from build123d import *

# Parameters (mm, degrees)
SKETCH2_R                 = 1.5
MAIN_EXTRUDE_DEPTH        = 21.5
HORIZONTAL_CUT_DEPTH      = 48.59062889
HORIZONTAL_CUT_DEPTH_BACK = 48.59062889
SKETCH5_OUTSIDE_W         = 47.542
SKETCH5_OUTSIDE_H         = 58.496
VERTICAL_CUT_DEPTH        = 15.063100578
END_FILLET_R              = 2
SPRING_PLACE_CUT_DEPTH    = 14
FILLET5_R                 = 10
FILLET4_R                 = 5
CUT_EXTRUDE1_DEPTH        = 52.882041504
CUT_EXTRUDE2_START        = -16.243126
CUT_EXTRUDE2_DEPTH        = 16.243126


# Read off the part's stored shape, not the designer's step: vertical-cut
with BuildPart() as part:
    # Sketch2 → main-extrude (new, symmetric)
    with BuildSketch(Plane.XY):
        with BuildLine():
            Line((26.046045858, 30.659682992), (19.902405526, 34.961506265))
            Line((19.902405526, 34.961506265), (11.298758981, 22.6742256))
            Line((11.298758981, 22.6742256), (1.690473047, 27.154642913))
            ThreePointArc((1.690473047, 27.154642913), (-2.003746596, 26.991347579), (-3.985523805, 23.869411765))
            Line((-3.985523805, 23.869411765), (-5.978285707, 0.51))
            ThreePointArc((-5.978285707, 0.51), (-1.419809226, -5.829591904), (5.543277195, -2.296100594))
            Line((5.543277195, -2.296100594), (7.669311717, -2.952527164))
            Line((7.669311717, -2.952527164), (7.722039638, 4.490290033))
            Line((7.722039638, 4.490290033), (26.046045858, 30.659682992))
        make_face()
        Circle(SKETCH2_R, mode=Mode.SUBTRACT)
        with Locations((0, 23.529411765)):
            Circle(SKETCH2_R, mode=Mode.SUBTRACT)
    extrude(amount=MAIN_EXTRUDE_DEPTH, both=True)

    # Sketch5 outside → horizontal-cut (cut, two sides: drawn at the far end of the back side and taken through both)
    with BuildSketch(Plane(origin=(0, 27.529411765, 0), x_dir=(-1, 0, 0), z_dir=(0, -1, 0)).offset(-HORIZONTAL_CUT_DEPTH_BACK)):
        with Locations((-10.023, 0)):
            Rectangle(SKETCH5_OUTSIDE_W, SKETCH5_OUTSIDE_H)
        Polygon((-5.543277195, -21.5), (6, -21.5), (6, 21.5), (-5.543277195, 21.5), (-7.669311717, 21.5), (-11.298758981, 7.5), (-26.046045858, 7.5), (-26.046045858, -7.5), (-11.298758981, -7.5), (-7.669311717, -21.5), align=None, mode=Mode.SUBTRACT)
    extrude(amount=HORIZONTAL_CUT_DEPTH + HORIZONTAL_CUT_DEPTH_BACK, mode=Mode.SUBTRACT)

    # vertical-cut outline → vertical-cut (cut)
    with BuildSketch(Plane(origin=(-1.956623805, 47.652438964, 0), x_dir=(0, 0, 1), z_dir=(0.9963809512430475, -0.08499999999999992, 0))):
        Polygon((10, 28.250815058), (10, 18), (21.5, 18), (21.5, 41.313669441), align=None)
        Polygon((-21.5, 18), (-10, 18), (-10, 28.250815058), (-21.5, 41.313669441), align=None)
    extrude(amount=VERTICAL_CUT_DEPTH, mode=Mode.SUBTRACT)

    # end-fillet
    end_fillet_edges = [part.edges().sort_by_distance(p)[0] for p in [
        (19.902405526, 34.961506265, 0),
        (26.046045858, 30.659682992, 0),
        (22.974225692, 32.810594628, 7.5),
        (22.974225692, 32.810594628, -7.5),
    ]]
    fillet(end_fillet_edges, radius=END_FILLET_R)

    # Sketch13 → spring-place-cut (cut, symmetric)
    with BuildSketch(Plane.XY):
        with BuildLine():
            Line((4.750311853, 13.645607612), (-4.788285707, 14.459333317))
            Line((-4.788285707, 14.459333317), (-5.468285707, 6.488285707))
            Line((-5.468285707, 6.488285707), (-5.978285707, 0.51))
            ThreePointArc((-5.978285707, 0.51), (-1.419809226, -5.829591904), (5.543277195, -2.296100594))
            Line((5.543277195, -2.296100594), (5.568173284, -2.303787419))
            Line((5.568173284, -2.303787419), (5.732956787, -1.770086573))
            ThreePointArc((5.732956787, -1.770086573), (5.96812639, -0.61763047), (5.973944242, 0.558560826))
            Line((5.973944242, 0.558560826), (4.750311853, 13.645607612))
        make_face()
    extrude(amount=SPRING_PLACE_CUT_DEPTH, both=True, mode=Mode.SUBTRACT)

    # Fillet5
    fillet5_edges = [part.edges().sort_by_distance(p)[0] for p in [
        (-0.018986927, 14.052470465, 14),
        (-0.018986927, 14.052470465, -14),
    ]]
    fillet(fillet5_edges, radius=FILLET5_R)

    # Fillet4
    # the kernel refuses this fillet: 5 mm, written as the material it adds along each edge
    with BuildSketch(Plane(origin=(11.298758981, 22.6742256, -17.98874539), x_dir=(-0.9063077870366477, 0.42261826174070405, 0), z_dir=(0, 0, 1))) as fillet4_piece_1_section:
        with BuildLine():
            CenterArc((FILLET4_R * 0.839099631177, -FILLET4_R), FILLET4_R, 90, 80)
            Line((-FILLET4_R * 0.145708121835, -FILLET4_R * 0.826351822333), (0, 0))
            Line((0, 0), (FILLET4_R * 0.839099631177, 0))
        make_face()
    fillet4_piece_1 = extrude(amount=25.48874539, mode=Mode.PRIVATE)
    fillet4_piece_1 = split(fillet4_piece_1, bisect_by=Plane(origin=(9.938648559, 23.630642265, -10), z_dir=(0, 0, 1)), keep=Keep.TOP, mode=Mode.PRIVATE)
    fillet4_piece_1 = split(fillet4_piece_1, bisect_by=Plane(origin=(10.933336463, 23.630642265, -8.909557674), z_dir=(-0.9679999612731994, 0, 0.25095034364408525)), keep=Keep.TOP, mode=Mode.PRIVATE)
    fillet4_piece_1 = split(fillet4_piece_1, bisect_by=Plane(origin=(9.938648559, 23.630642265, -7.5), z_dir=(0, 0, -1)), keep=Keep.TOP, mode=Mode.PRIVATE)
    add(fillet4_piece_1)
    with BuildSketch(Plane(origin=(11.298758981, 22.6742256, -7.5), x_dir=(-0.9063077870366477, 0.42261826174070405, 0), z_dir=(0, 0, 1))) as fillet4_piece_2_section:
        with BuildLine():
            CenterArc((FILLET4_R * 0.839099631177, -FILLET4_R), FILLET4_R, 90, 80)
            Line((-FILLET4_R * 0.145708121835, -FILLET4_R * 0.826351822333), (0, 0))
            Line((0, 0), (FILLET4_R * 0.839099631177, 0))
        make_face()
    fillet4_piece_2 = extrude(amount=15, mode=Mode.PRIVATE)
    fillet4_piece_2 = split(fillet4_piece_2, bisect_by=Plane(origin=(13.081425039, 23.673797808, 0.623656853), z_dir=(-0.9679999612731994, 0, -0.2509503436440852)), keep=Keep.TOP, mode=Mode.PRIVATE)
    fillet4_piece_2 = split(fillet4_piece_2, bisect_by=Plane(origin=(13.081425039, 23.673797808, -0.623656853), z_dir=(-0.9679999612731994, 0, 0.25095034364408525)), keep=Keep.TOP, mode=Mode.PRIVATE)
    add(fillet4_piece_2)
    with BuildSketch(Plane(origin=(11.298758981, 22.6742256, -7.5), x_dir=(-0.9063077870366477, 0.42261826174070405, 0), z_dir=(0, 0, 1))) as fillet4_piece_3_section:
        with BuildLine():
            CenterArc((FILLET4_R * 0.839099631177, -FILLET4_R), FILLET4_R, 90, 80)
            Line((-FILLET4_R * 0.145708121835, -FILLET4_R * 0.826351822333), (0, 0))
            Line((0, 0), (FILLET4_R * 0.839099631177, 0))
        make_face()
    fillet4_piece_3 = extrude(amount=15, mode=Mode.PRIVATE)
    fillet4_piece_3 = split(fillet4_piece_3, bisect_by=Plane(origin=(14.480371863, 24.591366471, -4.772552021), z_dir=(-0.9679999612731994, 0, -0.2509503436440852)), keep=Keep.TOP, mode=Mode.PRIVATE)
    fillet4_piece_3 = split(fillet4_piece_3, bisect_by=Plane(origin=(11.912432267, 24.591366471, -5.132855534), z_dir=(0.9679999612731994, 0, -0.25095034364408525)), keep=Keep.TOP, mode=Mode.PRIVATE)
    add(fillet4_piece_3)
    with BuildSketch(Plane(origin=(11.298758981, 22.6742256, -7.5), x_dir=(-0.9063077870366477, 0.42261826174070405, 0), z_dir=(0, 0, 1))) as fillet4_piece_4_section:
        with BuildLine():
            CenterArc((FILLET4_R * 0.839099631177, -FILLET4_R), FILLET4_R, 90, 80)
            Line((-FILLET4_R * 0.145708121835, -FILLET4_R * 0.826351822333), (0, 0))
            Line((0, 0), (FILLET4_R * 0.839099631177, 0))
        make_face()
    fillet4_piece_4 = extrude(amount=15, mode=Mode.PRIVATE)
    fillet4_piece_4 = split(fillet4_piece_4, bisect_by=Plane(origin=(11.912432267, 24.591366471, 5.132855534), z_dir=(0.9679999612731994, 0, 0.2509503436440852)), keep=Keep.TOP, mode=Mode.PRIVATE)
    fillet4_piece_4 = split(fillet4_piece_4, bisect_by=Plane(origin=(14.480371863, 24.591366471, 4.772552021), z_dir=(-0.9679999612731994, 0, 0.25095034364408525)), keep=Keep.TOP, mode=Mode.PRIVATE)
    add(fillet4_piece_4)
    with BuildSketch(Plane(origin=(11.298758981, 22.6742256, -7.5), x_dir=(-0.9063077870366477, 0.42261826174070405, 0), z_dir=(0, 0, 1))) as fillet4_piece_5_section:
        with BuildLine():
            CenterArc((FILLET4_R * 0.839099631177, -FILLET4_R), FILLET4_R, 90, 80)
            Line((-FILLET4_R * 0.145708121835, -FILLET4_R * 0.826351822333), (0, 0))
            Line((0, 0), (FILLET4_R * 0.839099631177, 0))
        make_face()
    fillet4_piece_5 = extrude(amount=25.48874539, mode=Mode.PRIVATE)
    fillet4_piece_5 = split(fillet4_piece_5, bisect_by=Plane(origin=(9.938648559, 23.630642265, 10), z_dir=(0, 0, -1)), keep=Keep.TOP, mode=Mode.PRIVATE)
    fillet4_piece_5 = split(fillet4_piece_5, bisect_by=Plane(origin=(10.933336463, 23.630642265, 8.909557674), z_dir=(-0.9679999612731994, 0, -0.2509503436440852)), keep=Keep.TOP, mode=Mode.PRIVATE)
    fillet4_piece_5 = split(fillet4_piece_5, bisect_by=Plane(origin=(9.938648559, 23.630642265, 7.5), z_dir=(0, 0, 1)), keep=Keep.TOP, mode=Mode.PRIVATE)
    add(fillet4_piece_5)
    with BuildSketch(Plane(origin=(11.298758981, 22.6742256, -7.5), x_dir=(-0.9063077870366477, 0.42261826174070405, 0), z_dir=(0, 0, 1))) as fillet4_piece_6_section:
        with BuildLine():
            CenterArc((FILLET4_R * 0.839099631177, -FILLET4_R), FILLET4_R, 90, 80)
            Line((-FILLET4_R * 0.145708121835, -FILLET4_R * 0.826351822333), (0, 0))
            Line((0, 0), (FILLET4_R * 0.839099631177, 0))
        make_face()
    fillet4_piece_6 = extrude(amount=15, mode=Mode.PRIVATE)
    fillet4_piece_6 = split(fillet4_piece_6, bisect_by=Plane(origin=(13.263621158, 25.832677019, -0.079134917), z_dir=(0.9679999612731994, 0, 0.2509503436440852)), keep=Keep.TOP, mode=Mode.PRIVATE)
    fillet4_piece_6 = split(fillet4_piece_6, bisect_by=Plane(origin=(13.263621158, 25.832677019, 0.079134917), z_dir=(0.9679999612731994, 0, -0.25095034364408525)), keep=Keep.TOP, mode=Mode.PRIVATE)
    add(fillet4_piece_6)

    # Sketch16 → Cut-Extrude1 (cut, through all)
    with BuildSketch(Plane(origin=(3.042409669, 35.663518124, 0), x_dir=(0.9963809512430474, -0.08499999999999996, 0), z_dir=(0.08499999999999996, 0.9963809512430474, 0))):
        with BuildLine():
            Line((18.345710894, -1.6), (10.345710894, -1.6))
            ThreePointArc((10.345710894, -1.6), (8.745710894, 0), (10.345710894, 1.6))
            Line((10.345710894, 1.6), (18.345710894, 1.6))
            ThreePointArc((18.345710894, 1.6), (19.945710894, 0), (18.345710894, -1.6))
        make_face()
    extrude(amount=-CUT_EXTRUDE1_DEPTH, mode=Mode.SUBTRACT)

    # Sketch17 → Cut-Extrude2 (cut)
    with BuildSketch(Plane(origin=(2.286753534, 26.80561955, 0), x_dir=(0.9963809512430474, -0.08499999999999996, 0), z_dir=(0.08499999999999996, 0.9963809512430474, 0)).offset(CUT_EXTRUDE2_START)):
        with BuildLine():
            Line((24.627792818, 3), (13.058532698, 3))
            ThreePointArc((13.058532698, 3), (10.058532698, 0), (13.058532698, -3))
            Line((13.058532698, -3), (24.627792818, -3))
            ThreePointArc((24.627792818, -3), (27.627792818, 0), (24.627792818, 3))
        make_face()
    extrude(amount=CUT_EXTRUDE2_DEPTH, mode=Mode.SUBTRACT)


solid = part.part
Check sheet for the modelled part. Datum: model origin and axes. Units: mm. A direction names the side the tool comes from. Give positions to 0.01 mm unless a question says otherwise; leave off trailing zeros. Loops run counter-clockwise (first coordinate to the right, second up) from the corner with the lowest first, then second, coordinate; pieces in that order, holes last. Notation, with made-up numbers: M -6,66.5 L 47,66.5 A18 cw 47,81.5 Z; hole C 53.5,8 d1. An arc over 180 degrees is marked long. Answer as a JSON object with one key per item and string values. Group by question number.
Q1. Material ranges on line 1 along Z through (x, y) = (4, 4); line 2 along Z through (x, y) = (19, 32); line 3 along Y through (x, z) = (0, -18), recorded low to high. Write a range as [from, to].
Q2. Release check for a two-part mould opening along X. For faces 4 (the flat face through (1, 2, -21.5)), 5 (the flat face through (5.37, 7.01, 0.2)), 6 (the cylindrical face through (-0.325, 22.065, -0.14)), 7 (the flat face through (17.774, 25.484, 2.146)) record: released by +X, released by -X, zero draft, split by the parting line, or undercut.
Q3. Cross-section at C-C on z = -15. Record the cut outline in (x, y).
Q4. Access from +Z, -Z, +X, -X, +Y, -Y to the whole of each face (thin tool, end or side, straight path). Record for faces 1 (the flat face through (17, 24, 7.5)), 2 (the cylindrical face through (5.966, -0.634, 0.196)), 3 (the flat face through (0.048, 14.047, 0.056)).
Q5. Cross-section at A-A on z = 12. Record the cut outline in (x, y), then the cut area to 3 significant figures.
Q6. Cross-section at B-B on y = 2.5. Record the cut outline in (x, z).
Q7. Go/stop test with flat-tipped pins: P1, Ø8.5, axis at x = 17.5, y = 19, coming from the +Z side; P2, Ø15, axis at x = 16.5, y = 24.5, coming from the -Z side; P3, Ø2.5, axis at x = 17.5, y = 31.5, coming from the -Z side. Record where each tip stops, or that it passes through.
Q8. Cross-section at D-D on x = 0.5. Give the number of separate pieces and of enclosed holes in the cut face, then the cut area to 3 significant figures.
Evaluation:
{
 "1": {"line 1": "z = [-21.5, -13.99], [13.99, 21.5]", "line 2": "z = [-7.5, -1.6], [1.6, 7.5]", "line 3": "y = [-6, -1.5], [1.5, 10.01]"},
 "2": {"face 4": "zero draft", "face 5": "released by -X", "face 6": "undercut", "face 7": "undercut"},
 "3": {"outline": "M -5.98,0.51 A6 ccw 5.54,-2.3 L 7.67,-2.95 L 7.72,4.49 L 9.35,6.82 L 9.35,12.63 L -4.84,13.84 Z; hole C 0,0 d3"},
 "4": {"face 1": "+Z, +X, +Y, -Y", "face 2": "-X", "face 3": "-X, -Y"},
 "5": {"outline": "M -5.13,10.47 L 5.13,9.6 L 5.97,0.56 A6 cw 5.73,-1.77 L 5.57,-2.3 L 7.67,-2.95 L 7.72,4.49 L 10.13,7.93 L 10.13,15.99 L -4.55,17.24 Z", "area": "135 mm2"},
 "6": {"outline": "M -5.81,-21.5 L 7.67,-21.5 L 7.71,-21.35 L 7.71,21.35 L 7.67,21.5 L -5.81,21.5 L -5.81,14 L 5.79,14 L 5.79,-14 L -5.81,-14 Z"},
 "7": {"P1": "stops at z = 7.5", "P2": "stops at z = -10", "P3": "stops at z = -7.5"},
 "8": {"separate pieces": "4", "enclosed holes": "0", "area": "480 mm2"}
}
